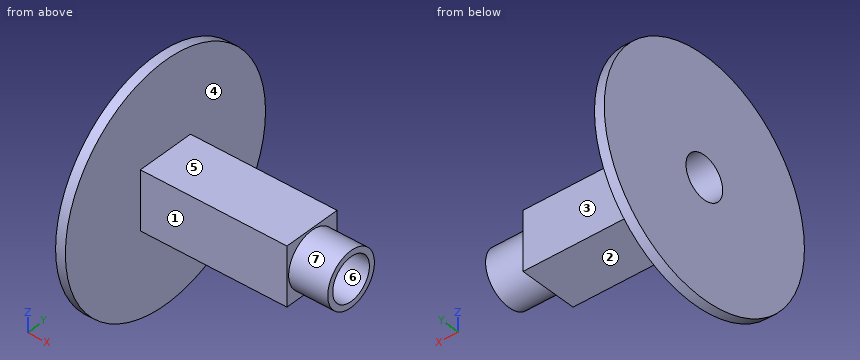
```python
from build123d import *

# Parameters (mm, degrees)
F0_R     = 14
F0_R_2   = 11
F1_DEPTH = 100
F0_W     = 30
F0_H     = 30
F2_DEPTH = 80
F0_R_3   = 60
F3_DEPTH = 5


with BuildPart() as f1:
    # F0 (on Right) → F1 (new body)
    with BuildSketch(Plane.YZ):
        Circle(F0_R)
        Circle(F0_R_2, mode=Mode.SUBTRACT)
    extrude(amount=F1_DEPTH)

    # F0 (on Right) → F2 (join)
    with BuildSketch(Plane.YZ):
        Rectangle(F0_W, F0_H)
        Circle(F0_R, mode=Mode.SUBTRACT)
    extrude(amount=F2_DEPTH)

    # F0 (on Right) → F3 (join)
    with BuildSketch(Plane.YZ):
        Circle(F0_R_3)
        Rectangle(F0_W, F0_H, mode=Mode.SUBTRACT)
    extrude(amount=F3_DEPTH)


solid = f1.part
```
Here's how the part is built. I have some questions about the finished solid (model axes, mm). Face numbers are marked on the shaded views. A direction names the side the tool comes from. Round coordinates to 2 decimals unless told otherwise and drop trailing zeros. Order: outer loops, then holes, each group sorted by start corner. A loop starts at its lowest first (then second) coordinate and runs counter-clockwise, first axis right, second up. Notation, with made-up numbers: M 56.25,-12.5 L 68.25,-12.5 A20 ccw 68.25,25.5 Z; hole C -37,-29.5 d5. An arc over 180 degrees is marked long. Answer in a Markdown table with one row per item.
Item 1: Imagine slicing it at C-C, the plane x = 68.5. Write out the boundary of the cut face in (y, z).
A:
| item | result |
|---|---|
| outline | M -15,-15 L 15,-15 L 15,15 L -15,15 Z; hole C 0,0 d22 |
Item 2: Imagine slicing it at D-D, the plane y = -31.5. Write out the boundary of the cut face in (x, z), and give its area (3 significant figures).
A:
| item | result |
|---|---|
| outline | M 0,-51.07 L 5,-51.07 L 5,51.07 L 0,51.07 Z |
| area | 511 mm2 |
Item 3: For the marked faces 1, 2 and 3, which set-ups out of +Z, -Z, +X, -X, +Y, -Y let a thin tool reach every point of the face, with its end or its side?
A:
| item | result |
|---|---|
| face 1 | +Z, -Z, +X, -Y |
| face 2 | -Z, +X, +Y, -Y |
| face 3 | +Z, -Z, +X, +Y |
Item 4: Thinking about a two-plate mould opening in Z: for the marked faces 4, 5, 6 and 7, which applies, +Z half, -Z half, draft (parallel to the pull), parting line (faces both ways), or undercut?
A:
| item | result |
|---|---|
| face 4 | draft |
| face 5 | +Z half |
| face 6 | undercut |
| face 7 | parting line |
Item 5: Imagine slicing it at A-A, the plane z = 0. Write out the boundary of the cut face in (x, y).
A:
| item | result |
|---|---|
| outline | M 0,-60 L 5,-60 L 5,-15 L 80,-15 L 80,-14 L 100,-14 L 100,-11 L 0,-11 Z; M 0,11 L 100,11 L 100,14 L 80,14 L 80,15 L 5,15 L 5,60 L 0,60 Z |
Item 6: I'm going to push flat-ended pins straight in: pin 1 (24 mm diameter, centred on x = 24.5, z = -5.5, fed in from -Y); pin 2 (6 mm diameter, centred on y = -5.5, z = 45, fed in from +X); pin 3 (5 mm diameter, centred on x = 69.5, y = 12.5, fed in from -Z); pin 4 (13 mm diameter, centred on y = 0, z = 0, fed in from +X). Where does each tip first touch, or does it pass through?
A:
| item | result |
|---|---|
| pin 1 | stops at y = -15 |
| pin 2 | stops at x = 5 |
| pin 3 | stops at z = -15 |
| pin 4 | passes through |
Item 7: If I drill on L1, parallel to Z at x = 40, y = 0; L2, parallel to X at y = -19, z = -55; L3, parallel to Z at x = 54.5, y = 14, over which ranges is the centre line in solid material (lowest first)? Write a range as from..to.
A:
| item | result |
|---|---|
| L1 | z = -15..-11, 11..15 |
| L2 | x = 0..5 |
| L3 | z = -15..15 |
